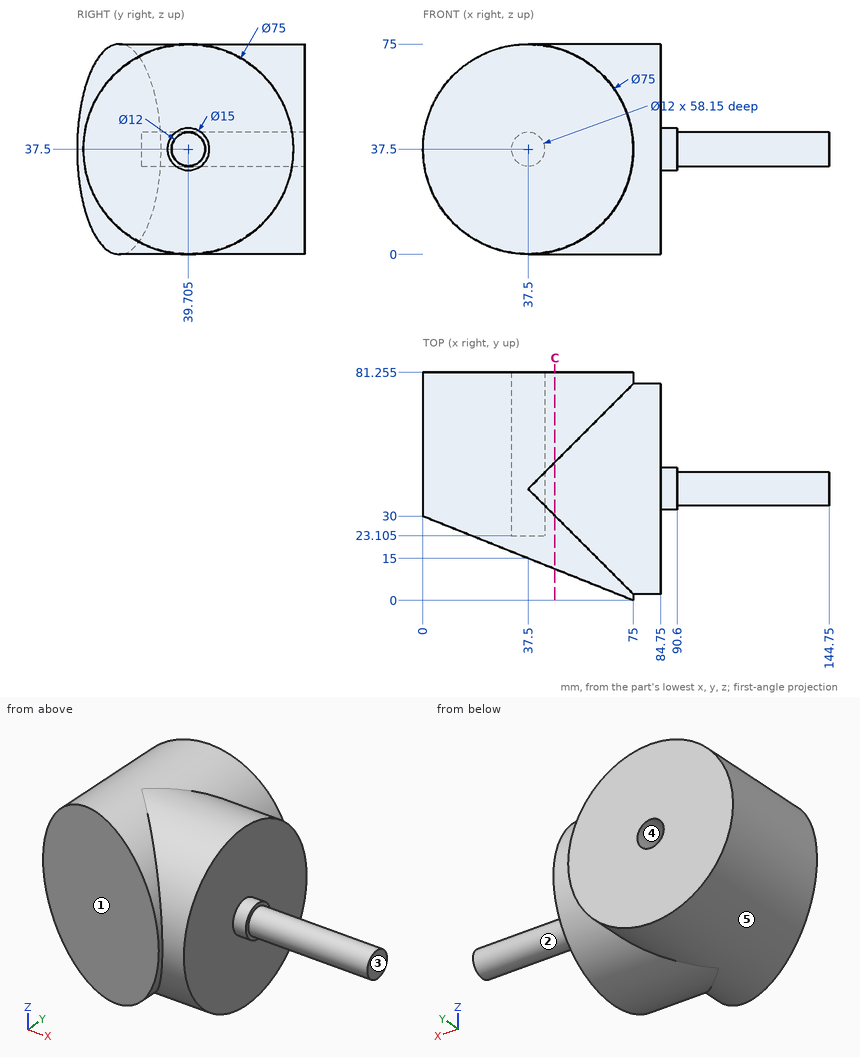
Input: dimensioned drawing with shaded views. Units: mm. Origin: part minimum x, y, z. A direction names the side the tool comes from. Coordinates: 2 decimals unless noted, no trailing zeros. Loops run counter-clockwise (first coordinate to the right, second up) from the corner with the lowest first, then second, coordinate; pieces in that order, holes last. Notation, with made-up numbers: M -16,-4.5 L 18,-4.5 A28 ccw 18,13.5 Z; hole C -30.75,6.25 d8. An arc over 180 degrees is marked long. Use a Markdown table: item, result. Add a question column.
Q1. First-contact query: pin 1 (1 mm diameter, centred on x = 68, y = 69, fed in from +Z); pin 2 (1 mm diameter, centred on x = 58, z = 56.5, fed in from -Y); pin 3 (12 mm diameter, centred on y = 13, z = 43.5, fed in from -X); pin 4 (5 mm diameter, centred on x = 88, y = 64, fed in from -Z). Flat tips, straight axial feed; report the tip coordinate or a pass-through.
Q2. Access query for the marked faces 1 and 2. Directions: +Z, -Z, +X, -X, +Y, -Y. A direction counts if a zero-diameter tool reaches every point of the face in a straight line with its end or side. Return the directions, or none.
Q3. Section query C-C, the plane x = 47. Return loops of the section in (y, z) (1 decimal).
Q4. Material intervals for L1, parallel to Z at x = 37, y = 36; L2, parallel to X at y = 48, z = 37; L3, parallel to X at y = 46, z = 37, sorted ascending.
Q5. Draft query along X for the marked faces 3, 4 and 5. Return one class per face: pulls with the +X half, pulls with the -X half, needs draft (parallel to the pull), parting line crosses it, or undercut.
Result:
| question | item | result |
|---|---|---|
| 1 | pin 1 | stops at z = 61.52 |
| 1 | pin 2 | stops at y = 6.6 |
| 1 | pin 3 | stops at x = 27.5 |
| 1 | pin 4 | passes through |
| 2 | face 1 | +Z, -Z, -X, -Y |
| 2 | face 2 | +X |
| 3 | outline | M 11.2,1.2 L 30.2,1.2 A37.5 ccw 49.2,1.2 L 81.3,1.2 L 81.3,73.8 L 49.2,73.8 A37.5 ccw 30.2,73.8 L 11.2,73.8 Z |
| 4 | L1 | z = 0 to 31.52, 43.48 to 75 |
| 4 | L2 | x = 0 to 31.52, 43.48 to 84.75 |
| 4 | L3 | x = 0 to 31.52, 43.48 to 90.6 |
| 5 | face 3 | pulls with the +X half |
| 5 | face 4 | undercut |
| 5 | face 5 | parting line crosses it |
